```python
from build123d import *

# Parameters (mm, degrees)
SKETCH1_R           = 1.35
SKETCH1_R_2         = 1.353883359
BOSS_EXTRUDE1_DEPTH = 2.5
BOSS_EXTRUDE2_DEPTH = 1
CHAMFER1_SIZE       = 1
CHAMFER2_SIZE       = 2.5


with BuildPart() as part:
    # Sketch1 → Boss-Extrude1 (new body)
    with BuildSketch(Plane.XY):
        with BuildLine():
            Line((-46.266968928, -27.305569911), (46.983031072, -27.305569911))
            ThreePointArc((46.983031072, -27.305569911), (52.736028884, -25.226770397), (55.831398017, -19.950684615))
            ThreePointArc((55.831398017, -19.950684615), (57.596036195, -0.805569911), (55.831398017, 18.339544793))
            ThreePointArc((55.831398017, 18.339544793), (52.736028884, 23.615630575), (46.983031072, 25.694430089))
            Line((46.983031072, 25.694430089), (-46.266968928, 25.694430089))
            ThreePointArc((-46.266968928, 25.694430089), (-52.019966741, 23.615630575), (-55.115335874, 18.339544793))
            ThreePointArc((-55.115335874, 18.339544793), (-56.879974052, -0.805569911), (-55.115335874, -19.950684615))
            ThreePointArc((-55.115335874, -19.950684615), (-52.019966741, -25.226770397), (-46.266968928, -27.305569911))
        make_face()
        with Locations((48.647296931, -19.366437107)):
            Circle(SKETCH1_R, mode=Mode.SUBTRACT)
        with Locations((48.647296931, 17.755297285)):
            Circle(SKETCH1_R, mode=Mode.SUBTRACT)
        with Locations((-47.931234788, 17.755297285)):
            Circle(SKETCH1_R, mode=Mode.SUBTRACT)
        with Locations((-47.931234788, -19.366437107)):
            Circle(SKETCH1_R_2, mode=Mode.SUBTRACT)
        with BuildLine():
            Line((-40.306968928, -14.970569911), (41.023031072, -14.970569911))
            ThreePointArc((41.023031072, -14.970569911), (44.558564977, -13.506103817), (46.023031072, -9.970569911))
            Line((46.023031072, -9.970569911), (46.023031072, 8.359430089))
            ThreePointArc((46.023031072, 8.359430089), (44.558564977, 11.894963995), (41.023031072, 13.359430089))
            Line((41.023031072, 13.359430089), (-40.306968928, 13.359430089))
            ThreePointArc((-40.306968928, 13.359430089), (-43.842502834, 11.894963995), (-45.306968928, 8.359430089))
            Line((-45.306968928, 8.359430089), (-45.306968928, -9.970569911))
            ThreePointArc((-45.306968928, -9.970569911), (-43.842502834, -13.506103817), (-40.306968928, -14.970569911))
        make_face(mode=Mode.SUBTRACT)
    extrude(amount=BOSS_EXTRUDE1_DEPTH)

    # Sketch2 → Boss-Extrude2 (add)
    with BuildSketch(Plane.XY.offset(2.5)):
        with BuildLine():
            Line((49.523031072, -9.970569911), (49.523031072, 8.359430089))
            ThreePointArc((49.523031072, 8.359430089), (47.033438712, 14.369837729), (41.023031072, 16.859430089))
            Line((41.023031072, 16.859430089), (-40.306968928, 16.859430089))
            ThreePointArc((-40.306968928, 16.859430089), (-46.317376569, 14.369837729), (-48.806968928, 8.359430089))
            Line((-48.806968928, 8.359430089), (-48.806968928, -9.970569911))
            ThreePointArc((-48.806968928, -9.970569911), (-46.317376569, -15.980977551), (-40.306968928, -18.470569911))
            Line((-40.306968928, -18.470569911), (41.023031072, -18.470569911))
            ThreePointArc((41.023031072, -18.470569911), (47.033438712, -15.980977551), (49.523031072, -9.970569911))
        make_face()
        with BuildLine():
            Line((41.023031072, 11.859430089), (-40.306968928, 11.859430089))
            ThreePointArc((-40.306968928, 11.859430089), (-42.781842663, 10.834303823), (-43.806968928, 8.359430089))
            Line((-43.806968928, 8.359430089), (-43.806968928, -9.970569911))
            ThreePointArc((-43.806968928, -9.970569911), (-42.781842663, -12.445443645), (-40.306968928, -13.470569911))
            Line((-40.306968928, -13.470569911), (41.023031072, -13.470569911))
            ThreePointArc((41.023031072, -13.470569911), (43.497904806, -12.445443645), (44.523031072, -9.970569911))
            Line((44.523031072, -9.970569911), (44.523031072, 8.359430089))
            ThreePointArc((44.523031072, 8.359430089), (43.497904806, 10.834303823), (41.023031072, 11.859430089))
        make_face(mode=Mode.SUBTRACT)
    extrude(amount=BOSS_EXTRUDE2_DEPTH)

    # Chamfer1
    chamfer1_edges = [part.edges().sort_by_distance(p)[0] for p in [
        (-42.781842663, 10.834303823, 3.5),
        (-43.806968928, -0.805569911, 3.5),
        (-42.781842663, -12.445443645, 3.5),
        (0.358031072, -13.470569911, 3.5),
        (43.497904806, -12.445443645, 3.5),
        (44.523031072, -0.805569911, 3.5),
        (43.497904806, 10.834303823, 3.5),
        (0.358031072, 11.859430089, 3.5),
        (49.523031072, -0.805569911, 3.5),
        (47.033438712, -15.980977551, 3.5),
        (0.358031072, -18.470569911, 3.5),
        (-46.317376569, -15.980977551, 3.5),
        (-48.806968928, -0.805569911, 3.5),
        (-46.317376569, 14.369837729, 3.5),
        (0.358031072, 16.859430089, 3.5),
        (47.033438712, 14.369837729, 3.5),
    ]]
    chamfer(chamfer1_edges, length=CHAMFER1_SIZE - 0.0001)  # a hair under: the kernel refuses the full size

    # Chamfer2
    chamfer2_edges = [part.edges().sort_by_distance(p)[0] for p in [
        (0.358031072, -27.305569911, 2.5),
        (52.736028884, -25.226770397, 2.5),
        (-52.019966741, -25.226770397, 2.5),
        (57.596036195, -0.805569911, 2.5),
        (-56.879974052, -0.805569911, 2.5),
        (52.736028884, 23.615630575, 2.5),
        (-52.019966741, 23.615630575, 2.5),
        (0.358031072, 25.694430089, 2.5),
    ]]
    chamfer(chamfer2_edges, length=CHAMFER2_SIZE - 0.0001)  # a hair under: the kernel refuses the full size


solid = part.part
```
Could you check a few things on this model? Use its own coordinates, in mm. A direction names the side the tool comes from. Round coordinates to 2 decimals unless told otherwise and drop trailing zeros. Order: outer loops, then holes, each group sorted by start corner. A loop starts at its lowest first (then second) coordinate and runs counter-clockwise, first axis right, second up. Notation, with made-up numbers: (8, -27.75) -> (56, -27.75) arc R10 ccw to (56, -11.75) -> close; hole circle Ø7 at (1, -2). An arc over 180 degrees is marked (long way). One line per question, with ' | ' between items.
Q1. If I drill on line 1 (X direction, y = -18.5, z = 0.65); line 2 (Z direction, x = 37, y = 22.5); line 3 (X direction, y = 4, z = 2.75), over which ranges is the centre line in solid material (lowest first)? Write a range as from..to.
Computed values:
line 1: -54.72..-48.97, -46.89..47.61, 49.68..55.43 | line 2: 0..2.5 | line 3: -48.56..-44.06, 44.77..49.27
Q2. I'm going to push flat-ended pins straight in: pin 1 (4 mm diameter, centred on x = -3, y = 10.5, fed in from -Z); pin 2 (2 mm diameter, centred on x = -12.5, z = 1.5, fed in from -Y); pin 3 (1.5 mm diameter, centred on y = 19, z = 2.5, fed in from -X); pin 4 (1.5 mm diameter, centred on x = 20, y = 10, fed in from +Z). Where does each tip first touch, or does it pass through?
Computed values:
pin 1: z = 2.5 | pin 2: y = -26.81 | pin 3: x = -53.18 | pin 4: through
Q3. We'd pull the mould along X, two halves only. Please class faces 4 (the face through (-45.663, 13.835, 3.34)), 5 (the face through (44.519, -13.545, 1.232)), 6 (the face through (0.1, 17.1, 2.5)): released by +X, released by -X, zero draft, split by the parting line, or undercut.
Computed values:
face 4: released by -X | face 5: undercut | face 6: zero draft
Q4. If we section it at B-B on z = 0.75: Write out the boundary of the cut face in (x, y).
Computed values:
outline: (-54.38, -19.81) arc R8.25 ccw to (-46.27, -26.56) -> (46.98, -26.56) arc R8.25 ccw to (55.09, -19.81) arc R103.99 ccw to (55.09, 18.2) arc R8.25 ccw to (46.98, 24.94) -> (-46.27, 24.94) arc R8.25 ccw to (-54.38, 18.2) arc R103.99 ccw to start; hole circle Ø2.71 at (-47.93, -19.37); hole circle Ø2.7 at (-47.93, 17.76); hole (-45.31, -9.97) arc R5 ccw to (-40.31, -14.97) -> (41.02, -14.97) arc R5 ccw to (46.02, -9.97) -> (46.02, 8.36) arc R5 ccw to (41.02, 13.36) -> (-40.31, 13.36) arc R5 ccw to (-45.31, 8.36) -> close; hole circle Ø2.7 at (48.65, -19.37); hole circle Ø2.7 at (48.65, 17.76)
Q5. Which directions (+Z, -Z, +X, -X, +Y, -Y) give clear straight access to the entire face, cutting with the end or side of a thin tool? Please do faces 1 (the face through (-43, -12.61, 2.77)), 2 (the face through (47.3, 17.8, 1.2)), 3 (the face through (-43.803, 11.934, 1.232)).
Computed values:
face 1: +Z | face 2: +Z, -Z | face 3: -Z
